from build123d import *

# Parameters (mm, degrees)
F2_R     = 5
F3_DEPTH = 2
F4_SIZE  = 0.1


# Not quite as in the source:
# - a fillet or chamfer that OpenCascade refuses, or shapes differently, is made with other operations: its cross-section is extruded or revolved along the edge and cut away or added


with BuildPart() as f1:
    # F0 (on Front) → F1 (revolve)
    with BuildSketch(Plane.XZ):
        Polygon((0, 3), (0, 0), (5, 0), (5, 3), (3, 6.4998515683), (1.38, 6.4998515683), (1.38, 3), align=None)
    revolve(axis=Axis((0, 0, 4.7499257841), (0, 0, 1)))

    # F2
    f2_edges = [f1.edges().sort_by_distance(p)[0] for p in [
        (-5, 0, 3),
    ]]
    fillet(f2_edges, radius=F2_R)

    # F3 (add): a face of the model
    f3_faces = [f1.faces().sort_by_distance(p)[0] for p in [
        (-2.9151471863, 0, 6.4998515683),
    ]]
    extrude(f3_faces, amount=F3_DEPTH)

    # F4
    f4_edges = [f1.edges().sort_by_distance(p)[0] for p in [
        (-1.38, 0, 8.499852),
    ]]
    chamfer(f4_edges, length=F4_SIZE)

    # F5: fillet of radius 35 on 1 edges, made by hand

    # F5_s1 → F5_t2 (revolve, cut)
    with BuildSketch(Plane.XZ):
        with BuildLine():
            ThreePointArc((1.48, 8.4998515683), (1.405008935, 7.1788664105), (1.38, 5.8559907549))
            Line((1.38, 5.8559907549), (1.38, 8.3998515683))
            Line((1.38, 8.3998515683), (1.48, 8.4998515683))
        make_face()
    revolve(axis=Axis((0, 0, 8.3998515683), (0, 0, 1)), mode=Mode.SUBTRACT)

    # F6: fillet of radius 7.9 on 1 edges, made by hand

    # F6_s1 → F6_t2 (revolve)
    with BuildSketch(Plane.XZ):
        with BuildLine():
            ThreePointArc((3, 8.4998515683), (3.276921402, 6.5233668652), (4.0403288808, 4.6793532357))
            Line((4.0403288808, 4.6793532357), (3, 6.4998515683))
            Line((3, 6.4998515683), (3, 8.4998515683))
        make_face()
    revolve(axis=Axis((0, 0, 6.4998515683), (0, 0, 1)))


solid = f1.part
Input: part model. Units: mm. Frame: model coordinates. A direction names the side the tool comes from. Round coordinates to 2 decimals unless told otherwise and drop trailing zeros. Order: outer loops, then holes, each group sorted by start corner. A loop starts at its lowest first (then second) coordinate and runs counter-clockwise, first axis right, second up. Notation, with made-up numbers: (-40, 83.25) - (1, 83.25) arc R10 cw to (1, 101.25) - close; hole circle Ø5 at (-3, -7). An arc over 180 degrees is marked (long way). Answer as a JSON object with one key per item and string values. Group by question number.
(1) Cut plane C-C (z = 5.5). Return loops of the section in (x, y).
(2) Pin query (flat end, axial travel): P1, Ø5, axis at y = -1, z = 6, coming from the +X side; P2, Ø1, axis at y = 3.5, z = 5, coming from the -X side. Return the tip coordinate at first contact, or that it passes through.
(3) Material intervals for probe 1 along Z at (x, y) = (0, -0.75); probe 2 along Y at (x, z) = (0, 3.8); probe 3 along X at (y, z) = (-1.25, 3.5), sorted ascending. Write a range as from..to.
(4) Reachability of faces 1 (the face through (0, 0, 3)), 2 (the face through (0, 0, 0)) from +Z, -Z, +X, -X, +Y, -Y: full face, straight path, thin tool, end or side. Return the list, or none.
(5) Cut plane B-B (z = 1). Return loops of the section in (x, y).
(6) Cut plane A-A (z = 7.75). Return loops of the section in (x, y), then the cut area to 3 significant figures.
(7) Draft query along Y for faces 3 (the face through (3, 4, 1)), 4 (the face through (1.3, -1.3, 8.5)), 5 (the face through (-0.299, -1.347, 4.408)). Return one class per face: released by +Y, released by -Y, zero draft, split by the parting line, or undercut.
Here are the results:
{
 "1": {"outline": "circle Ø7.27 at (0, 0); hole circle Ø2.76 at (0, 0)"},
 "2": {"P1": "stops at x = 4.61", "P2": "stops at x = -2.57"},
 "3": {"probe 1": "z = 0..3", "probe 2": "y = -4.52..-1.38, 1.38..4.52", "probe 3": "x = -4.48..-0.58, 0.58..4.48"},
 "4": {"face 1": "+Z", "face 2": "-Z, +X, -X, +Y, -Y"},
 "5": {"outline": "circle Ø10 at (0, 0)"},
 "6": {"outline": "circle Ø6.09 at (0, 0); hole circle Ø2.86 at (0, 0)", "area": "22.7 mm^2"},
 "7": {"face 3": "split by the parting line", "face 4": "zero draft", "face 5": "undercut"}
}
